Geometry: see drawing. Coordinates: mm, zero at the bounding-box minimum. Give positions to 0.01 mm unless a question says otherwise; leave off trailing zeros. Write each loop counter-clockwise with the first axis right and the second up, starting at its lowest first coordinate (ties: lowest second). Pieces come first, ordered by that corner, then holes. Notation, with made-up numbers: (7.25, 70.5) - (44.25, 70.5) arc R25 ccw to (44.25, 103.5) - close; hole circle Ø8 at (81.25, 54). An arc over 180 degrees is marked (long way). One line per question, with ' | ' between items. Start each with the question number.
(1) Pin query (flat end, axial travel): pin 1 (18 mm diameter, centred on x = 26.5, y = 32, fed in from +Z). Return the tip coordinate at first contact, or that it passes through.
(2) Ray query, line 1 (Z direction, x = 47, y = 22.5). Return the intervals inside material, ascending. Write a range as [from, to].
(3) Section A-A, the plane y = 21.5. Return loops of the section in (x, z), plus the area to 3 significant figures.
(4) Section B-B, the plane x = 20. Return loops of the section in (y, z), plus the area to 3 significant figures.
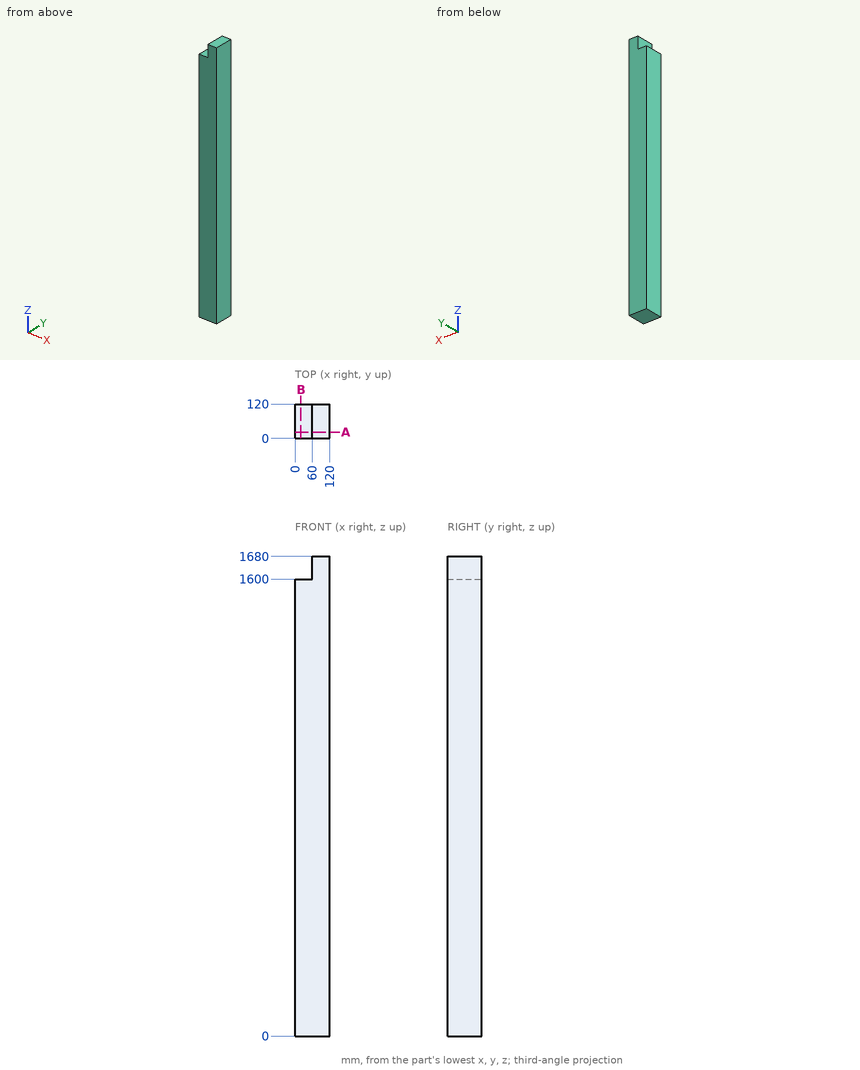
Check sheet entries:
1) pin 1: z = 1600
2) line 1: [0, 1600]
3) outline: (0, 0) - (120, 0) - (120, 1680) - (60, 1680) - (60, 1600) - (0, 1600) - close | area: 197,000 mm²
4) outline: (0, 0) - (120, 0) - (120, 1600) - (0, 1600) - close | area: 192,000 mm²
